CAD build for the part. Positions are in the model's coordinates, mm. Round coordinates to 2 decimals unless told otherwise and drop trailing zeros. Write each loop counter-clockwise with the first axis right and the second up, starting at its lowest first coordinate (ties: lowest second). Pieces come first, ordered by that corner, then holes. Notation, with made-up numbers: (27, -12.5) - (84, -12.5) arc R26 ccw to (84, 7.5) - close; hole circle Ø8 at (42, 3.25). An arc over 180 degrees is marked (long way). Put each result on its own line as item: value. Start each with the question number.
Item 1: Pin check, flat tips, straight feed: pin 1 Ø4.5 at (x, y) = (13.5, -7) entering from +Z; pin 2 Ø0.8 at (y, z) = (3.5, -0.5) entering from +X; pin 3 Ø1.2 at (x, z) = (4.5, -1) entering from +Y. Stop position of each tip, or through.
Item 2: Drill centre lines: line 1 (X direction, y = -7, z = -0.7); line 2 (Y direction, x = 13.5, z = -0.95); line 3 (X direction, y = 5.5, z = -0.95). Where is each one in solid material? Low to high. Write a range as from..to.
Item 3: Cut at D-D (y = 2.25). Give the cut face in (x, z).
Item 4: Cut at C-C (x = 13.5). Give the cut face in (y, z), and give its area (3 significant figures).
Item 5: Cut at A-A (y = -7). Give the cut face in (x, z), and give its area (3 significant figures).
Item 6: Cut at B-B (z = -0.4). Give the cut face in (x, y), and give its area (3 significant figures).
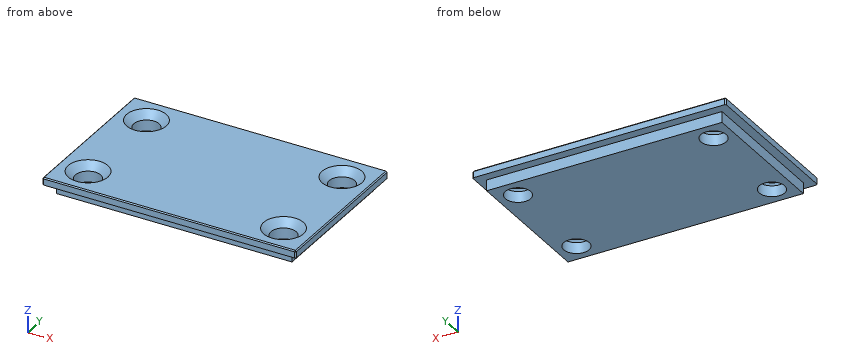
```python
from build123d import *

# Parameters (mm, degrees)
F0_W     = 35
F0_H     = 22
F1_DEPTH = 1
F2_SIZE  = 0.15
F3_W     = 32.5
F3_H     = 19.5
F4_DEPTH = 1.5
F5_R     = 1.75
F6_DEPTH = 25
F7_SIZE  = 1


with BuildPart() as f1:
    # F0 (on Top) → F1 (new body)
    with BuildSketch(Plane.XY):
        Rectangle(F0_W, F0_H)
    extrude(amount=F1_DEPTH)

    # F2
    f2_edges = [f1.edges().sort_by_distance(p)[0] for p in [
        (-17.5, 0, 1),
        (0, 11, 1),
        (17.5, 0, 1),
        (0, -11, 1),
        (-17.5, 11, 0.5),
        (17.5, 11, 0.5),
        (17.5, -11, 0.5),
        (-17.5, -11, 0.5),
    ]]
    chamfer(f2_edges, length=F2_SIZE)

    # F3 (on face) → F4 (join)
    with BuildSketch(Plane(origin=(0, 0, 0), x_dir=(1, 0, 0), z_dir=(0, 0, -1))):
        Rectangle(F3_W, F3_H)
    extrude(amount=F4_DEPTH)

    # F5 (on face) → F6 (cut)
    with BuildSketch(Plane(origin=(0, 0, -1.5), x_dir=(1, 0, 0), z_dir=(0, 0, -1))):
        with Locations((-13.5, 7)):
            Circle(F5_R)
        with Locations((-13.5, -7)):
            Circle(F5_R)
        with Locations((13.5, -7)):
            Circle(F5_R)
        with Locations((13.5, 7)):
            Circle(F5_R)
    extrude(amount=-F6_DEPTH, mode=Mode.SUBTRACT)

    # F7
    f7_edges = [f1.edges().sort_by_distance(p)[0] for p in [
        (-15.25, 7, 1),
        (11.75, 7, 1),
        (11.75, -7, 1),
        (-15.25, -7, 1),
    ]]
    chamfer(f7_edges, length=F7_SIZE)


solid = f1.part
```
Output values:
1. pin 1: z = 0.5
1. pin 2: x = 16.25
1. pin 3: y = 9.75
2. line 1: -16.25..-15.25, -11.75..11.75, 15.25..16.25
2. line 2: -9.75..-8.75, -5.25..5.25, 8.75..9.75
2. line 3: -16.25..-14.4, -12.6..12.6, 14.4..16.25
3. outline: (-17.5, 0) - (-16.25, 0) - (-16.25, -1.5) - (16.25, -1.5) - (16.25, 0) - (17.5, 0) - (17.5, 0.85) - (17.35, 1) - (-17.35, 1) - (-17.5, 0.85) - close
4. outline: (-11, 0) - (-9.75, 0) - (-9.75, -1.5) - (-8.75, -1.5) - (-8.75, 0) - (-9.75, 1) - (-10.85, 1) - (-11, 0.85) - close; (-5.25, -1.5) - (5.25, -1.5) - (5.25, 0) - (4.25, 1) - (-4.25, 1) - (-5.25, 0) - close; (8.75, -1.5) - (9.75, -1.5) - (9.75, 0) - (11, 0) - (11, 0.85) - (10.85, 1) - (9.75, 1) - (8.75, 0) - close
4. area: 31.7 mm2
5. outline: (-17.5, 0) - (-16.25, 0) - (-16.25, -1.5) - (-15.25, -1.5) - (-15.25, 0) - (-16.25, 1) - (-17.35, 1) - (-17.5, 0.85) - close; (-11.75, -1.5) - (11.75, -1.5) - (11.75, 0) - (10.75, 1) - (-10.75, 1) - (-11.75, 0) - close; (15.25, -1.5) - (16.25, -1.5) - (16.25, 0) - (17.5, 0) - (17.5, 0.85) - (17.35, 1) - (16.25, 1) - (15.25, 0) - close
5. area: 64.2 mm2
6. outline: (-16.25, -9.75) - (16.25, -9.75) - (16.25, 9.75) - (-16.25, 9.75) - close; hole circle Ø3.5 at (-13.5, -7); hole circle Ø3.5 at (-13.5, 7); hole circle Ø3.5 at (13.5, -7); hole circle Ø3.5 at (13.5, 7)
6. area: 595 mm2
